The listing builds one solid part. Answer for the finished solid, in the listing's coordinates (mm). A direction names the side the tool comes from. Coordinates: 2 decimals unless noted, no trailing zeros. Put each result on its own line as item: value. Start each with the question number.
```python
from build123d import *

# Parameters (mm, degrees)
AUFSATZ_LINEAR_AUSTRAGEN1_DEPTH      = 10
SKIZZE2_R                            = 2.175
SCHNITT_LINEAR_AUSTRAGEN1_DEPTH      = 8
SCHNITT_LINEAR_AUSTRAGEN2_DEPTH      = 30
SCHNITT_LINEAR_AUSTRAGEN2_DEPTH_BACK = 10
SKIZZE3_R                            = 2.3
VERRUNDUNG1_R                        = 2
VERRUNDUNG2_R                        = 0.2
VERRUNDUNG3_R                        = 0.5
FASE1_SIZE                           = 0.75
FASE2_SIZE                           = 0.4


with BuildPart() as part:
    # Skizze1 → Aufsatz-Linear austragen1 (new body)
    with BuildSketch(Plane.XY):
        with BuildLine():
            Line((10.15, 0), (10.15, -20.3))
            Line((10.15, -20.3), (-10.15, -20.3))
            Line((-10.15, -20.3), (-10.15, 0))
            Line((-10.15, 0), (-49.95, 0))
            Line((-49.95, 0), (-49.95, -20))
            ThreePointArc((-49.95, -20), (-25.317447047, -26.210871087), (0, -28.3))
            ThreePointArc((0, -28.3), (25.317447047, -26.210871087), (49.95, -20))
            Line((49.95, -20), (49.95, 0))
            Line((49.95, 0), (10.15, 0))
        make_face()
        with BuildLine():
            Line((17.15, -6), (17.15, -21.30603648))
            ThreePointArc((17.15, -21.30603648), (28.637839253, -19.511539955), (39.95, -16.823476023))
            Line((39.95, -16.823476023), (39.95, -6))
            Line((39.95, -6), (17.15, -6))
        make_face(mode=Mode.SUBTRACT)
        with BuildLine():
            Line((-17.15, -6), (-39.95, -6))
            Line((-39.95, -6), (-39.95, -16.823476023))
            ThreePointArc((-39.95, -16.823476023), (-28.637839253, -19.511539955), (-17.15, -21.30603648))
            Line((-17.15, -21.30603648), (-17.15, -6))
        make_face(mode=Mode.SUBTRACT)
    extrude(amount=AUFSATZ_LINEAR_AUSTRAGEN1_DEPTH)

    # Skizze2 → Schnitt-Linear austragen1 (cut)
    with BuildSketch(Plane(origin=(49.95, 0, 0), x_dir=(0, 0, -1), z_dir=(1, 0, 0))):
        with Locations((-5, -7)):
            Circle(SKIZZE2_R)
    schnitt_linear_austragen1 = extrude(amount=-SCHNITT_LINEAR_AUSTRAGEN1_DEPTH, mode=Mode.SUBTRACT)

    # Spiegeln1: Schnitt-Linear austragen1 across plane
    add(schnitt_linear_austragen1.mirror(Plane(origin=(0, 0, 0), x_dir=(0, 0, 1), z_dir=(1, 0, 0))), mode=Mode.SUBTRACT)

    # Skizze3 → Schnitt-Linear austragen2 (cut, two sides: drawn at the far end of the back side and taken through both)
    with BuildSketch(Plane.ZY.offset(-10.15).offset(-SCHNITT_LINEAR_AUSTRAGEN2_DEPTH_BACK)):
        with Locations(Location((5, -10.15, 0), (0, 0, 270))):
            Circle(SKIZZE3_R)
    extrude(amount=SCHNITT_LINEAR_AUSTRAGEN2_DEPTH + SCHNITT_LINEAR_AUSTRAGEN2_DEPTH_BACK, mode=Mode.SUBTRACT)

    # Verrundung1
    verrundung1_edges = [part.edges().sort_by_distance(p)[0] for p in [
        (49.95, 0, 5),
        (49.95, -20, 5),
        (-49.95, -20, 5),
        (-49.95, 0, 5),
        (-10.15, 0, 5),
        (10.15, 0, 5),
        (39.95, -16.823476023, 5),
        (39.95, -6, 5),
        (17.15, -21.30603648, 5),
        (-17.15, -21.30603648, 5),
        (-39.95, -6, 5),
        (-39.95, -16.823476023, 5),
    ]]
    fillet(verrundung1_edges, radius=VERRUNDUNG1_R)

    # Verrundung2
    verrundung2_edges = [part.edges().sort_by_distance(p)[0] for p in [
        (-10.15, -20.3, 5),
        (10.15, -20.3, 5),
    ]]
    fillet(verrundung2_edges, radius=VERRUNDUNG2_R)

    # Verrundung3
    verrundung3_edges = [part.edges().sort_by_distance(p)[0] for p in [
        (17.15, -6, 5),
        (-17.15, -6, 5),
    ]]
    fillet(verrundung3_edges, radius=VERRUNDUNG3_R)

    # Fase1
    fase1_edges = [part.edges().sort_by_distance(p)[0] for p in [
        (-17.831485792, -20.546408723, 0),
        (-17.831485792, -20.546408723, 10),
        (-39.536902903, -16.514831798, 0),
        (-39.536902903, -16.514831798, 10),
        (-39.364213562, -6.585786438, 0),
        (-39.364213562, -6.585786438, 10),
        (39.364213562, -6.585786438, 0),
        (39.364213562, -6.585786438, 10),
        (39.536902903, -16.514831798, 0),
        (39.536902903, -16.514831798, 10),
        (17.831485792, -20.546408723, 0),
        (17.831485792, -20.546408723, 10),
        (-10.15, -11.05, 0),
        (-10.15, -11.05, 10),
        (0, -20.3, 0),
        (0, -20.3, 10),
        (-10.091421356, -20.241421356, 0),
        (-10.091421356, -20.241421356, 10),
        (10.091421356, -20.241421356, 0),
        (10.091421356, -20.241421356, 10),
        (-27.8, -6, 10),
        (-27.8, -6, 0),
        (17.15, -12.771286766, 10),
        (17.15, -12.771286766, 0),
        (-17.296446609, -6.146446609, 0),
        (-17.296446609, -6.146446609, 10),
        (17.296446609, -6.146446609, 0),
        (17.296446609, -6.146446609, 10),
        (30.05, 0, 0),
        (30.05, 0, 10),
        (49.95, -10.281445763, 0),
        (0, -28.3, 0),
        (-49.95, -10.281445763, 0),
        (-30.05, 0, 0),
        (10.15, -11.05, 0),
        (29.00206817, -19.439458054, 0),
        (39.95, -11.648782352, 0),
        (27.8, -6, 0),
        (-29.00206817, -19.439458054, 0),
        (-17.15, -12.771286766, 0),
        (-39.95, -11.648782352, 0),
        (49.571435511, -19.733765937, 0),
        (-49.571435511, -19.733765937, 0),
        (-49.364213562, -0.585786438, 0),
        (-10.735786438, -0.585786438, 0),
        (10.735786438, -0.585786438, 0),
        (49.364213562, -0.585786438, 0),
        (49.95, -10.281445763, 10),
        (39.95, -11.648782352, 10),
        (29.00206817, -19.439458054, 10),
        (27.8, -6, 10),
        (10.15, -11.05, 10),
        (-30.05, 0, 10),
        (-49.95, -10.281445763, 10),
        (0, -28.3, 10),
        (-17.15, -12.771286766, 10),
        (-29.00206817, -19.439458054, 10),
        (-39.95, -11.648782352, 10),
        (49.571435511, -19.733765937, 10),
        (-49.571435511, -19.733765937, 10),
        (-49.364213562, -0.585786438, 10),
        (-10.735786438, -0.585786438, 10),
        (10.735786438, -0.585786438, 10),
        (49.364213562, -0.585786438, 10),
    ]]
    chamfer(fase1_edges, length=FASE1_SIZE)

    # Fase2
    fase2_edges = [part.edges().sort_by_distance(p)[0] for p in [
        (49.95, -7, 7.175),
        (-49.95, -7, 7.175),
    ]]
    chamfer(fase2_edges, length=FASE2_SIZE)


solid = part.part
```
1) Given pin 1 Ø4 at (x, y) = (-21, -7.5) entering from -Z; pin 2 Ø1.3 at (y, z) = (-7.5, 5.5) entering from -X; pin 3 Ø2 at (x, z) = (-0.5, 6.5) entering from +Y, each flat-ended and moving along its own axis, determine where each tip first touches the part or whether it passes through.
2) Straight lines are drawn through the part: probe 1 along Y at (x, z) = (-15, 5); probe 2 along X at (y, z) = (-7, 4.5); probe 3 along Z at (x, y) = (12.25, -10.15). For each, find the intervals that lie inside material, in ascending order.
3) For faces 5 (the face through (-10.72, -0.6, 5.06)), 6 (the face through (11.076, -0.902, 9.714)), 7 (the face through (-13.601, -8.325, 3.6)), determine the directions among +Z, -Z, +X, -X, +Y, -Y from which every point of the face is accessible in a straight line to the end or side of a thin tool.
4) Determine the mould class of faces 1 (the face through (39.56, -6.36, 9.55)), 2 (the face through (49.06, -0.92, 0.3)), 3 (the face through (0, -20.3, 5)), 4 (the face through (30, 0, 5)) for opening direction X: +X half, -X half, draft (parallel to the pull), parting line (faces both ways), or undercut.
Answers follow:
1. pin 1: stops at z = 0.25
1. pin 2: stops at x = -41.95
1. pin 3: stops at y = -20.3
2. probe 1: y = -27.57 to -12.45, -7.85 to 0
2. probe 2: x = -41.95 to -39.68, -17.15 to -10.15, 10.15 to 17.15, 39.68 to 41.95
2. probe 3: z = 0 to 2.7, 7.3 to 10
3. face 5: +Z, -Z, +Y
3. face 6: +Z, +Y
3. face 7: none
4. face 1: undercut
4. face 2: +X half
4. face 3: undercut
4. face 4: draft
